Here's how the part is built. I have some questions about the finished solid (model axes, mm). A direction names the side the tool comes from. Round coordinates to 2 decimals unless told otherwise and drop trailing zeros. Order: outer loops, then holes, each group sorted by start corner. A loop starts at its lowest first (then second) coordinate and runs counter-clockwise, first axis right, second up.
```python
from build123d import *

# Parameters (mm, degrees)
SKETCH1_R                  = 9
SKETCH1_R_2                = 6
MAIN_DEPTH                 = 9.5
SKETCH2_W                  = 40
SKETCH2_H                  = 19
SKETCH2_R                  = 4
SKETCH2_R_2                = 1.35
BALLSUPPORTEXTRUSION_DEPTH = 5
SKETCH3_R                  = 5.15
BALLSUPPORTHOLE_DEPTH      = 4
FILLET2_R                  = 2
SKETCH5_R                  = 6
CUT_EXTRUDE2_DEPTH         = 20
SKETCH6_W                  = 12.514718626
SKETCH6_H                  = 11
CUT_EXTRUDE3_DEPTH         = 15
FILLET3_R                  = 1
FILLET4_R                  = 6


with BuildPart() as part:
    # Sketch1 → Main (new body, symmetric)
    with BuildSketch(Plane.XY):
        Circle(SKETCH1_R)
        Circle(SKETCH1_R_2, mode=Mode.SUBTRACT)
    extrude(amount=MAIN_DEPTH, both=True)

    # Sketch2 → BallSupportExtrusion (add, symmetric)
    with BuildSketch(Plane(origin=(0, 0, 0), x_dir=(1, 0, 0), z_dir=(0, 1, 0))):
        with Locations((20, 0)):
            Rectangle(SKETCH2_W, SKETCH2_H)
        with Locations((33, 0)):
            Circle(SKETCH2_R, mode=Mode.SUBTRACT)
        with Locations((33, 7)):
            Circle(SKETCH2_R_2, mode=Mode.SUBTRACT)
        with Locations((33, -7)):
            Circle(SKETCH2_R_2, mode=Mode.SUBTRACT)
    extrude(amount=BALLSUPPORTEXTRUSION_DEPTH, both=True)

    # Sketch3 → BallSupportHole (cut)
    with BuildSketch(Plane(origin=(0, 5, 0), x_dir=(1, 0, 0), z_dir=(0, 1, 0))):
        with Locations((33, 0)):
            Circle(SKETCH3_R)
    ballsupporthole = extrude(amount=-BALLSUPPORTHOLE_DEPTH, mode=Mode.SUBTRACT)

    # Fillet2
    fillet2_edges = [part.edges().sort_by_distance(p)[0] for p in [
        (7.483314774, 5, 0),
    ]]
    fillet(fillet2_edges, radius=FILLET2_R)

    # Sketch5 → Cut-Extrude2 (cut, through all)
    with BuildSketch(Plane.XY.offset(9.5)):
        Circle(SKETCH5_R)
    extrude(amount=-CUT_EXTRUDE2_DEPTH, mode=Mode.SUBTRACT)

    # Mirror1: BallSupportHole across plane
    add(ballsupporthole.mirror(Plane.ZX), mode=Mode.SUBTRACT)

    # Sketch6 → Cut-Extrude3 (cut, through all)
    with BuildSketch(Plane(origin=(0, 5, 0), x_dir=(1, 0, 0), z_dir=(0, 1, 0))):
        with Locations((18.742640687, 0)):
            Rectangle(SKETCH6_W, SKETCH6_H)
    extrude(amount=-CUT_EXTRUDE3_DEPTH, mode=Mode.SUBTRACT)

    # Fillet3
    fillet3_edges = [part.edges().sort_by_distance(p)[0] for p in [
        (12.485281374, 0, 5.5),
        (12.485281374, 0, -5.5),
        (25, 0, -5.5),
        (25, 0, 5.5),
    ]]
    fillet(fillet3_edges, radius=FILLET3_R)

    # Fillet4
    fillet4_edges = [part.edges().sort_by_distance(p)[0] for p in [
        (40, 0, 9.5),
        (40, 0, -9.5),
    ]]
    fillet(fillet4_edges, radius=FILLET4_R)


solid = part.part
```
1) If we section it at D-D (x = 33): Write out the boundary of the cut face in (y, z).
2) If we section it at B-B (y = 0): Write out the boundary of the cut face in (x, z), plus the area to 3 significant figures.
3) If we section it at A-A (z = 0): Write out the boundary of the cut face in (x, y).
4) We'd pull the mould along X, two halves only. Please class faces 1 (the cylindrical face through (32.824, -0.07, -8.339)), 2 (the flat face through (27.5, 5, -0.1)), 3 (the cylindrical face through (38.289, 0.07, 7.696)): +X half, -X half, draft (parallel to the pull), parting line (faces both ways), or undercut.
5) I need wall thicknesses on line 1 (X direction, y = 0.25, z = 0.25); line 2 (Z direction, x = 33, y = -2.25); line 3 (X direction, y = -2.5, z = -7). Which ranges of each line are inside material? Lowest first, please.
6) For faces 4 (the cylindrical face through (27.855, 3.028, -0.226)), 5 (the cylindrical face through (27.855, -3.028, -0.226)), 6 (the flat face through (19, 0, 5.5)), which set-ups out of +Z, -Z, +X, -X, +Y, -Y let a thin tool reach every point of the face, with its end or its side?
7) I'm going to push flat-ended pins straight in: pin 1 (5 mm diameter, centred on x = 33.5, z = -2, fed in from -Y); pin 2 (1.5 mm diameter, centred on x = 31, z = 6.5, fed in from -Y); pin 3 (8 mm diameter, centred on x = 34, z = 0, fed in from +Y). Where does each tip first touch, or does it pass through?
8) If we section it at C-C (x = 0): Write out the boundary of the cut face in (y, z), plus the area to 3 significant figures.
Solutions:
1. outline: (-5, -9.5) - (5, -9.5) - (5, -8.35) - (-5, -8.35) - close; (-5, -5.65) - (5, -5.65) - (5, -5.15) - (1, -5.15) - (1, -4) - (-1, -4) - (-1, -5.15) - (-5, -5.15) - close; (-5, 5.15) - (-1, 5.15) - (-1, 4) - (1, 4) - (1, 5.15) - (5, 5.15) - (5, 5.65) - (-5, 5.65) - close; (-5, 8.35) - (5, 8.35) - (5, 9.5) - (-5, 9.5) - close
2. outline: (-9, -9.5) - (-6, -9.5) - (-6, 9.5) - (-9, 9.5) - close; (6, -9.5) - (34, -9.5) arc R6 ccw to (40, -3.5) - (40, 3.5) arc R6 ccw to (34, 9.5) - (6, 9.5) - close; hole (12.49, -4.5) arc R1 ccw to (13.49, -5.5) - (24, -5.5) arc R1 ccw to (25, -4.5) - (25, 4.5) arc R1 ccw to (24, 5.5) - (13.49, 5.5) arc R1 ccw to (12.49, 4.5) - close; hole circle Ø8 at (33, 0); hole circle Ø2.7 at (33, -7); hole circle Ø2.7 at (33, 7)
2. area: 489 mm2
3. outline: (6.94, 5.73) arc R9 ccw (long way) to (7.48, -5) - (12.49, -5) - (12.49, 5) - (8.49, 5) arc R2 cw to start; (25, -5) - (27.85, -5) - (27.85, -1) - (29, -1) - (29, 1) - (27.85, 1) - (27.85, 5) - (25, 5) - close; (37, -1) - (38.15, -1) - (38.15, -5) - (40, -5) - (40, 5) - (38.15, 5) - (38.15, 1) - (37, 1) - close; hole circle Ø12 at (0, 0)
4. face 1: undercut
4. face 2: draft
4. face 3: +X half
5. line 1: x = -9 to -5.99, 5.99 to 12.49, 25 to 29.01, 36.99 to 40
5. line 2: z = -9.5 to -8.35, -5.65 to -5.15, 5.15 to 5.65, 8.35 to 9.5
5. line 3: x = -8.65 to -5.45, 5.45 to 31.65, 34.35 to 38.87
6. face 4: +Y
6. face 5: -Y
6. face 6: +Y, -Y
7. pin 1: stops at y = -1
7. pin 2: stops at y = -5
7. pin 3: stops at y = 1
8. outline: (-9, -9.5) - (-6, -9.5) - (-6, 9.5) - (-9, 9.5) - close; (6, -9.5) - (9, -9.5) - (9, 9.5) - (6, 9.5) - close
8. area: 114 mm2
